```python
from build123d import *

# Parameters (mm, degrees)
SKETCH1_R           = 1.4732
BOSS_EXTRUDE1_DEPTH = 3


with BuildPart() as part:
    # Sketch1 → Boss-Extrude1 (new body)
    with BuildSketch(Plane(origin=(0, 0, 0), x_dir=(1, 0, 0), z_dir=(0, 1, 0))):
        with BuildLine():
            Line((-33.75, 25.45), (-31.41, 25.45))
            Line((-31.41, 25.45), (-31.41, 31.5))
            ThreePointArc((-31.41, 31.5), (-31.336776695, 31.676776695), (-31.16, 31.75))
            Line((-31.16, 31.75), (53, 31.75))
            ThreePointArc((53, 31.75), (55.121320344, 30.871320344), (56, 28.75))
            Line((56, 28.75), (56, -28.75))
            ThreePointArc((56, -28.75), (55.121320344, -30.871320344), (53, -31.75))
            Line((53, -31.75), (-53.2, -31.75))
            ThreePointArc((-53.2, -31.75), (-55.321320344, -30.871320344), (-56.2, -28.75))
            Line((-56.2, -28.75), (-56.2, -20.85))
            ThreePointArc((-56.2, -20.85), (-56.126776695, -20.673223305), (-55.95, -20.6))
            Line((-55.95, -20.6), (-50, -20.6))
            Line((-50, -20.6), (-50, -8.9))
            Line((-50, -8.9), (-55.95, -8.9))
            ThreePointArc((-55.95, -8.9), (-56.126776695, -8.826776695), (-56.2, -8.65))
            Line((-56.2, -8.65), (-56.2, 7.15))
            ThreePointArc((-56.2, 7.15), (-56.126776695, 7.326776695), (-55.95, 7.4))
            Line((-55.95, 7.4), (-50, 7.4))
            Line((-50, 7.4), (-50, 19.1))
            Line((-50, 19.1), (-55.95, 19.1))
            ThreePointArc((-55.95, 19.1), (-56.126776695, 19.173223305), (-56.2, 19.35))
            Line((-56.2, 19.35), (-56.2, 28.75))
            ThreePointArc((-56.2, 28.75), (-55.321320344, 30.871320344), (-53.2, 31.75))
            Line((-53.2, 31.75), (-43.34, 31.75))
            ThreePointArc((-43.34, 31.75), (-43.163223305, 31.676776695), (-43.09, 31.5))
            Line((-43.09, 31.5), (-43.09, 25.45))
            Line((-43.09, 25.45), (-40.75, 25.45))
            ThreePointArc((-40.75, 25.45), (-40.573223305, 25.376776695), (-40.5, 25.2))
            Line((-40.5, 25.2), (-40.5, 20.35))
            Line((-40.5, 20.35), (-34, 20.35))
            Line((-34, 20.35), (-34, 25.2))
            ThreePointArc((-34, 25.2), (-33.926776695, 25.376776695), (-33.75, 25.45))
        make_face()
        with Locations(Location((-47, 21.25, 0), (0, 0, 270))):
            Circle(SKETCH1_R, mode=Mode.SUBTRACT)
        with Locations(Location((-47, -22.75, 0), (0, 0, 270))):
            Circle(SKETCH1_R, mode=Mode.SUBTRACT)
        with Locations(Location((47, -22.75, 0), (0, 0, 270))):
            Circle(SKETCH1_R, mode=Mode.SUBTRACT)
        with Locations(Location((47, 21.25, 0), (0, 0, 270))):
            Circle(SKETCH1_R, mode=Mode.SUBTRACT)
        with BuildLine():
            Line((-52.699999734, -6.75), (-50.699999734, -6.75))
            ThreePointArc((-50.699999734, -6.75), (-49.84644625, -7.103553297), (-50.2, -6.25))
            Line((-50.2, -6.25), (-50.2, 4.749999991))
            ThreePointArc((-50.2, 4.749999991), (-49.846447452, 5.603553619), (-50.700000632, 5.25))
            Line((-50.700000632, 5.25), (-52.700000632, 5.25))
            ThreePointArc((-52.700000632, 5.25), (-53.553554237, 5.603553165), (-53.2, 4.75))
            Line((-53.2, 4.75), (-53.2, -6.25))
            ThreePointArc((-53.2, -6.25), (-53.553553031, -7.103553485), (-52.699999734, -6.75))
        make_face(mode=Mode.SUBTRACT)
        with BuildLine():
            Line((-28.2, 28.249999625), (-28.2, 26.249999625))
            ThreePointArc((-28.2, 26.249999625), (-28.553553309, 25.396446153), (-27.7, 25.749999854))
            Line((-27.7, 25.749999854), (-12.7, 25.749999854))
            ThreePointArc((-12.7, 25.749999854), (-11.846446528, 25.396446775), (-12.2, 26.250000084))
            Line((-12.2, 26.250000084), (-12.2, 28.250000084))
            ThreePointArc((-12.2, 28.250000084), (-11.846446639, 29.103553504), (-12.7, 28.75))
            Line((-12.7, 28.75), (-27.7, 28.75))
            ThreePointArc((-27.7, 28.75), (-28.553553523, 29.103552882), (-28.2, 28.249999625))
        make_face(mode=Mode.SUBTRACT)
        with BuildLine():
            Line((20, 28.249999625), (20, 26.249999625))
            ThreePointArc((20, 26.249999625), (19.646446691, 25.396446153), (20.5, 25.749999854))
            Line((20.5, 25.749999854), (35.5, 25.749999854))
            ThreePointArc((35.5, 25.749999854), (36.353553472, 25.396446775), (36, 26.250000084))
            Line((36, 26.250000084), (36, 28.250000084))
            ThreePointArc((36, 28.250000084), (36.353553361, 29.103553504), (35.5, 28.75))
            Line((35.5, 28.75), (20.5, 28.75))
            ThreePointArc((20.5, 28.75), (19.646446477, 29.103552882), (20, 28.249999625))
        make_face(mode=Mode.SUBTRACT)
        with BuildLine():
            Line((-36.2, -26.250000146), (-36.2, -28.250000146))
            ThreePointArc((-36.2, -28.250000146), (-36.553553309, -29.103553617), (-35.7, -28.749999916))
            Line((-35.7, -28.749999916), (-20.7, -28.749999916))
            ThreePointArc((-20.7, -28.749999916), (-19.846446528, -29.103552995), (-20.2, -28.249999686))
            Line((-20.2, -28.249999686), (-20.2, -26.249999686))
            ThreePointArc((-20.2, -26.249999686), (-19.846446639, -25.396446266), (-20.7, -25.74999977))
            Line((-20.7, -25.74999977), (-35.7, -25.74999977))
            ThreePointArc((-35.7, -25.74999977), (-36.553553523, -25.396446888), (-36.2, -26.250000146))
        make_face(mode=Mode.SUBTRACT)
        with BuildLine():
            Line((20, -26.250000146), (20, -28.250000146))
            ThreePointArc((20, -28.250000146), (19.646446691, -29.103553617), (20.5, -28.749999916))
            Line((20.5, -28.749999916), (35.5, -28.749999916))
            ThreePointArc((35.5, -28.749999916), (36.353553472, -29.103552995), (36, -28.249999686))
            Line((36, -28.249999686), (36, -26.249999686))
            ThreePointArc((36, -26.249999686), (36.353553361, -25.396446266), (35.5, -25.74999977))
            Line((35.5, -25.74999977), (20.5, -25.74999977))
            ThreePointArc((20.5, -25.74999977), (19.646446477, -25.396446888), (20, -26.250000146))
        make_face(mode=Mode.SUBTRACT)
        with BuildLine():
            Line((50.500000146, -21.75), (52.500000146, -21.75))
            ThreePointArc((52.500000146, -21.75), (53.353553617, -22.103553309), (52.999999916, -21.25))
            Line((52.999999916, -21.25), (52.999999916, -6.25))
            ThreePointArc((52.999999916, -6.25), (53.353552995, -5.396446528), (52.499999686, -5.75))
            Line((52.499999686, -5.75), (50.499999686, -5.75))
            ThreePointArc((50.499999686, -5.75), (49.646446266, -5.396446639), (49.99999977, -6.25))
            Line((49.99999977, -6.25), (49.99999977, -21.25))
            ThreePointArc((49.99999977, -21.25), (49.646446888, -22.103553523), (50.500000146, -21.75))
        make_face(mode=Mode.SUBTRACT)
        with BuildLine():
            Line((50.500000146, 5.75), (52.500000146, 5.75))
            ThreePointArc((52.500000146, 5.75), (53.353553617, 5.396446691), (52.999999916, 6.25))
            Line((52.999999916, 6.25), (52.999999916, 21.25))
            ThreePointArc((52.999999916, 21.25), (53.353552995, 22.103553472), (52.499999686, 21.75))
            Line((52.499999686, 21.75), (50.499999686, 21.75))
            ThreePointArc((50.499999686, 21.75), (49.646446266, 22.103553361), (49.99999977, 21.25))
            Line((49.99999977, 21.25), (49.99999977, 6.25))
            ThreePointArc((49.99999977, 6.25), (49.646446888, 5.396446477), (50.500000146, 5.75))
        make_face(mode=Mode.SUBTRACT)
    extrude(amount=BOSS_EXTRUDE1_DEPTH)


solid = part.part
```
Input: part model. Units: mm. Frame: model coordinates. A direction names the side the tool comes from. Round coordinates to 2 decimals unless told otherwise and drop trailing zeros. Write each loop counter-clockwise with the first axis right and the second up, starting at its lowest first coordinate (ties: lowest second). Pieces come first, ordered by that corner, then holes. Notation, with made-up numbers: (25, 41) - (29, 41) arc R27 cw to (29, 61) - close; hole circle Ø9 at (27, 56.5). An arc over 180 degrees is marked (long way). Write item = value, one per line.
(1) Pull-direction query (X, two-part tool) for faces 1 (the flat face through (50, 1, 14)), 2 (the flat face through (1, 0, 0)), 3 (the cylindrical face through (55.14, 1.48, 30.85)), 4 (the flat face through (52, 1, 5.75)); classes: +X half, -X half, draft (parallel to the pull), parting line (faces both ways), or undercut.
Geometry check:
face_1 = undercut
face_2 = draft
face_3 = +X half
face_4 = undercut
(2) Section query B-B on z = 14. Output: boundary loops of the cut face in (x, y), then the cut area to 3 significant figures.
Geometry check:
outline = (-50, 0) - (50, 0) - (50, 3) - (-50, 3) - close; (53, 0) - (56, 0) - (56, 3) - (53, 3) - close
area = 309 mm^2
(3) Section query D-D on y = 1.85. State how many separate pieces and enclosed holes the cut face has, then the cut area to 3 significant figures.
Geometry check:
separate_pieces = 1
enclosed_holes = 11
area = 6,500 mm^2
(4) Section query A-A on x = -47. Output: boundary loops of the cut face in (y, z).
Geometry check:
outline = (0, -31.75) - (3, -31.75) - (3, -22.72) - (0, -22.72) - close; (0, -19.78) - (3, -19.78) - (3, 21.28) - (0, 21.28) - close; (0, 24.22) - (3, 24.22) - (3, 31.75) - (0, 31.75) - close
(5) Material intervals for probe 1 along Z at (x, y) = (23, 2.2); probe 2 along X at (y, z) = (2.5, 20); probe 3 along X at (y, z) = (0.9, -25), sorted ascending.
Geometry check:
probe_1 = -31.75 to -28.75, -25.75 to 25.75, 28.75 to 31.75
probe_2 = -50 to 50, 53 to 56
probe_3 = -56.2 to -40.5, -34 to 56
(6) Section query C-C on z = 1.5. Output: boundary loops of the cut face in (x, y), then the cut area to 3 significant figures.
Geometry check:
outline = (-56.2, 0) - (-53.2, 0) - (-53.2, 3) - (-56.2, 3) - close; (-50.2, 0) - (56, 0) - (56, 3) - (-50.2, 3) - close
area = 328 mm^2
(7) Access query for faces 5 (the flat face through (-34, 1, -23)), 6 (the flat face through (51, 1, 21.75)), 7 (the flat face through (-50, 1, 15)). Directions: +Z, -Z, +X, -X, +Y, -Y. A direction counts if a zero-diameter tool reaches every point of the face in a straight line with its end or side. Return the directions, or none.
Geometry check:
face_5 = -Z, +Y, -Y
face_6 = +Y, -Y
face_7 = -X, +Y, -Y
(8) Contact query for flat-ended pins moving along their axis: pin 1 Ø1.8 at (x, z) = (-47, -21.25) entering from +Y; pin 2 Ø0.9 at (y, z) = (1.5, 13) entering from -X; pin 3 Ø1.5 at (x, y) = (-36.5, 1) entering from -Z. Output: stop coordinate, or through.
Geometry check:
pin_1 = through
pin_2 = -50
pin_3 = -20.35
